from build123d import *

# Parameters (mm, degrees)
SKETCH1_W           = 35.4
SKETCH1_H           = 35.4
SKETCH1_W_2         = 25.475
SKETCH1_H_2         = 25.475
BOSS_EXTRUDE1_DEPTH = 50.0375
SKETCH1_3_W         = 35.4
SKETCH1_3_H         = 35.4
SKETCH1_3_W_2       = 25.475
SKETCH1_3_H_2       = 25.475
BOSS_EXTRUDE2_DEPTH = 9.9625
SKETCH2_R           = 4.05
BOSS_EXTRUDE5_DEPTH = 35.4
SKETCH3_R           = 3.15
CUT_EXTRUDE1_DEPTH  = 88.31496149
SKETCH4_R           = 5.5
CUT_EXTRUDE2_DEPTH  = 25.6125
SKETCH5_R           = 7
SKETCH5_R_2         = 4.05
BOSS_EXTRUDE6_DEPTH = 0.5
BOSS_EXTRUDE7_DEPTH = 5
CUT_EXTRUDE3_REACH  = 69.006
SKETCH7_R           = 2.8


with BuildPart() as part:
    # Sketch1 → Boss-Extrude1 (new body)
    with BuildSketch(Plane(origin=(0, 0, 0), x_dir=(1, 0, 0), z_dir=(0, 1, 0))):
        Rectangle(SKETCH1_W, SKETCH1_H)
        Rectangle(SKETCH1_W_2, SKETCH1_H_2, mode=Mode.SUBTRACT)
    extrude(amount=BOSS_EXTRUDE1_DEPTH)

    # Sketch1<3> → Boss-Extrude2 (add)
    # profile 1 of 2: a face of its own
    with BuildSketch(Plane(origin=(0, 0, 0), x_dir=(1, 0, 0), z_dir=(0, 1, 0))):
        Rectangle(SKETCH1_3_W, SKETCH1_3_H)
        Rectangle(SKETCH1_3_W_2, SKETCH1_3_H_2, mode=Mode.SUBTRACT)
    # profile 2 of 2: a face of its own
    with BuildSketch(Plane(origin=(0, 0, 0), x_dir=(1, 0, 0), z_dir=(0, 1, 0))):
        Rectangle(SKETCH1_3_W_2, SKETCH1_3_H_2)
    extrude(amount=-BOSS_EXTRUDE2_DEPTH)

    # Sketch2 → Boss-Extrude5 (add)
    with BuildSketch(Plane.XY.offset(-17.7)):
        with BuildLine():
            Line((-17.7, -15.9125), (-17.7, -9.9625))
            Line((-17.7, -9.9625), (17.7, -9.9625))
            Line((17.7, -9.9625), (17.7, -15.9125))
            ThreePointArc((17.7, -15.9125), (0, -33.6125), (-17.7, -15.9125))
        make_face()
        with Locations(Location((0, -15.9625, 0), (0, 0, 180))):
            Circle(SKETCH2_R, mode=Mode.SUBTRACT)
    extrude(amount=BOSS_EXTRUDE5_DEPTH)

    # Sketch3 → Cut-Extrude1 (cut, through all)
    with BuildSketch(Plane(origin=(0, -33.6125, 0), x_dir=(-1, 0, 0), z_dir=(0, -1, 0))):
        with Locations(Location((0, 0, 0), (0, 0, 90))):
            Circle(SKETCH3_R)
    extrude(amount=-CUT_EXTRUDE1_DEPTH, mode=Mode.SUBTRACT)

    # Sketch4 → Cut-Extrude2 (cut)
    with BuildSketch(Plane(origin=(0, -33.6125, 0), x_dir=(-1, 0, 0), z_dir=(0, -1, 0))):
        with Locations(Location((0, 0, 0), (0, 0, 90))):
            Circle(SKETCH4_R)
    extrude(amount=-CUT_EXTRUDE2_DEPTH, mode=Mode.SUBTRACT)

    # Sketch5 → Boss-Extrude6 (add)
    with BuildSketch(Plane.XY.offset(17.7)):
        with Locations(Location((0, -15.9625, 0), (0, 0, 180))):
            Circle(SKETCH5_R)
        with Locations(Location((0, -15.9625, 0), (0, 0, 180))):
            Circle(SKETCH5_R_2, mode=Mode.SUBTRACT)
    boss_extrude6 = extrude(amount=BOSS_EXTRUDE6_DEPTH)

    # Mirror1: Boss-Extrude6 across plane
    add(boss_extrude6.mirror(Plane.XY))

    # Sketch6 → Boss-Extrude7 (add)
    with BuildSketch(Plane.XY.offset(17.7)):
        Polygon((0, 4.583434556), (17.7, 14.802534321), (17.7, 50.0375), (-17.7, 50.0375), (-17.7, 14.802534321), align=None)
    boss_extrude7 = extrude(amount=BOSS_EXTRUDE7_DEPTH)

    # Sketch7 → Cut-Extrude3 (cut, up to next)
    with BuildSketch(Plane.XY.offset(22.7), mode=Mode.PRIVATE) as cut_extrude3_sk1:
        with Locations((0, 20.0375)):
            Circle(SKETCH7_R)
    cut_extrude3_tool1 = extrude(cut_extrude3_sk1.sketch, amount=-CUT_EXTRUDE3_REACH, mode=Mode.PRIVATE) & part.part
    cut_extrude3 = cut_extrude3_tool1.solids().sort_by_distance((0, 20.0375, 22.7))[0]
    add(cut_extrude3, mode=Mode.SUBTRACT)

    # Mirror2: Boss-Extrude7, Cut-Extrude3 across plane
    add(boss_extrude7.mirror(Plane.XY))
    add(cut_extrude3.mirror(Plane.XY), mode=Mode.SUBTRACT)


solid = part.part
Input: part model. Units: mm. Frame: model coordinates. A direction names the side the tool comes from. Round coordinates to 2 decimals unless told otherwise and drop trailing zeros. Loops run counter-clockwise (first coordinate to the right, second up) from the corner with the lowest first, then second, coordinate; pieces in that order, holes last. Notation, with made-up numbers: (20, 46) -> (62, 46) arc R19 cw to (62, 79) -> close; hole circle Ø10 at (76.25, 16). An arc over 180 degrees is marked (long way). Answer as a JSON object with one key per item and string values. Group by question number.
1) Section query A-A on z = 0. Output: boundary loops of the cut face in (x, y), plus the area to 3 significant figures.
2) Draft query along Y for faces 4 (the cylindrical face through (-3.863, -17.179, 10.859)), 5 (the flat face through (0, 25, -12.738)), 6 (the cylindrical face through (0.911, -22.903, -17.946)), 7 (the flat face through (3, 0, -3)). Return one class per face: +Y half, -Y half, draft (parallel to the pull), parting line (faces both ways), or undercut.
3) Section query D-D on z = 14. Output: boundary loops of the cut face in (x, y).
4) Section query C-C on z = -10.5. Output: boundary loops of the cut face in (x, y).
5) Ray query, L1, parallel to Y at x = 0, z = -17; L2, parallel to X at y = 46.5, z = -10; L3, parallel to Y at x = 0, z = -18. Return the intervals inside material, ascending.
6) Section query B-B on x = -9. Output: boundary loops of the cut face in (y, z), plus the area to 3 significant figures.
7) Reachability of faces 1 (the flat face through (-4, -9, 17.7)), 2 (the flat face through (-3, -13, 18.2)), 3 (the flat face through (-12.738, 25, 0)) from +Z, -Z, +X, -X, +Y, -Y: full face, straight path, thin tool, end or side. Return the list, or none.
8) Pin query (flat end, axial travel): pin 1 (4 mm diameter, centred on x = 6, z = -1.5, fed in from +Y); pin 2 (15.5 mm diameter, centred on x = -3, y = -15, fed in from +Z); pin 3 (5.5 mm diameter, centred on x = 0.5, z = -2, fed in from -Y); pin 4 (5 mm diameter, centred on x = 0, z = 0, fed in from -Y). Return the tip coordinate at first contact, or that it passes through.
Reply:
{
 "1": {"outline": "(-17.7, -15.91) arc R17.7 ccw to (-5.5, -32.74) -> (-5.5, -8) -> (-3.15, -8) -> (-3.15, 0) -> (-12.74, 0) -> (-12.74, 50.04) -> (-17.7, 50.04) -> close; (3.15, -8) -> (5.5, -8) -> (5.5, -32.74) arc R17.7 ccw to (17.7, -15.91) -> (17.7, 50.04) -> (12.74, 50.04) -> (12.74, 0) -> (3.15, 0) -> close", "area": "1,220 mm2"},
 "2": {"face 4": "undercut", "face 5": "draft", "face 6": "undercut", "face 7": "+Y half"},
 "3": {"outline": "(-17.7, -15.91) arc R17.7 ccw to (17.7, -15.91) -> (17.7, 50.04) -> (-17.7, 50.04) -> close; hole circle Ø8.1 at (0, -15.96); hole circle Ø5.6 at (0, 20.04)"},
 "4": {"outline": "(-17.7, -15.91) arc R17.7 ccw to (17.7, -15.91) -> (17.7, 50.04) -> (12.74, 50.04) -> (12.74, 0) -> (-12.74, 0) -> (-12.74, 50.04) -> (-17.7, 50.04) -> close; hole circle Ø8.1 at (0, -15.96)"},
 "5": {"L1": "y = -33.61 to -20.01, -11.91 to 17.24, 22.84 to 50.04", "L2": "x = -17.7 to -12.74, 12.74 to 17.7", "L3": "y = -22.96 to -20.01, -11.91 to -8.96, 4.58 to 17.24, 22.84 to 50.04"},
 "6": {"outline": "(-31.15, -17.7) -> (9.78, -17.7) -> (9.78, -22.7) -> (50.04, -22.7) -> (50.04, -12.74) -> (0, -12.74) -> (0, 12.74) -> (50.04, 12.74) -> (50.04, 22.7) -> (9.78, 22.7) -> (9.78, 17.7) -> (-31.15, 17.7) -> close", "area": "2,000 mm2"},
 "7": {"face 1": "+Z", "face 2": "+Z, +X, -X, -Y", "face 3": "+Y"},
 "8": {"pin 1": "stops at y = 0", "pin 2": "stops at z = 18.2", "pin 3": "stops at y = -8", "pin 4": "passes through"}
}
